Autodesk Inventor part; units mm, degrees
ref_plane "YZ Plane" through (0, 0, 0) normal (1, 0, 0) x (0, 1, 0)
ref_plane "XZ Plane" through (0, 0, 0) normal (0, 1, 0) x (-1, 0, 0)
ref_plane "XY Plane" through (0, 0, 0) normal (0, 0, 1) x (1, 0, 0)
sketch "Sketch1" plane through (0, 0, 0) normal (0, 1, 0) x (-1, 0, 0)
  line L0 (0, 0) -> (-70, 0)
  line L1 (-70, 0) -> (-70, -50)
  line L2 (-70, -50) -> (0, -50)
  line L3 (0, -50) -> (0, 0)
  line L4 (0, -50) -> (0, -67.7966)
  line L5 (0, -67.7966) -> (-70, -50)
  dimension "d0" = 70
  dimension "d1" = 50
  dimension "d45" = 14.264
extrude "Extrusion1" add sketch "Sketch1" along normal blind 6
sketch "Sketch2" plane through (0, 6, 0) normal (0, 1, 0) x (1, 0, 0)
  line L0 (70, 50) -> (58.37, 52.9568) construction
  line L1 (70, 50) -> (0, 67.7966) construction
  line L2 (58.37, 52.9568) -> (52.555, 54.4352)
  line L3 (52.555, 54.4352) -> (53.2942, 57.3427)
  line L4 (53.2942, 57.3427) -> (59.1092, 55.8643)
  line L5 (59.1092, 55.8643) -> (58.37, 52.9568)
  line L6 (23.4799, 61.8271) -> (17.6649, 63.3055)
  line L7 (17.6649, 63.3055) -> (18.4041, 66.213)
  line L8 (18.4041, 66.213) -> (24.2191, 64.7346)
  line L9 (24.2191, 64.7346) -> (23.4799, 61.8271)
  point P0 (0, 0)
  dimension "d9" = 12
  dimension "d10" = 6
  dimension "d11" = 3
  dimension "d15" = 6
  dimension "d16" = 3
  dimension "d17" = 30
extrude "Extrusion2" add sketch "Sketch2" against normal blind 6
sketch "Sketch3" plane through (0, 6, 0) normal (0, 1, 0) x (1, 0, 0)
  line L0 (70, 0) -> (70, 50)
  line L1 (70, 54) -> (64, 54)
  line L2 (64, 54) -> (64, 41)
  line L3 (64, 41) -> (70, 41)
  line L4 (70, 41) -> (70, 54)
  line L5 (70, 0) -> (64, 0)
  line L6 (64, 0) -> (64, 9)
  line L7 (64, 9) -> (70, 9)
  line L8 (70, 9) -> (70, 0)
  line L9 (70, 35) -> (64, 35)
  line L10 (64, 35) -> (64, 15)
  line L11 (64, 15) -> (70, 15)
  line L12 (70, 15) -> (70, 35)
  point P0 (0, 0)
  dimension "d18" = 6
  dimension "d20" = 6
  dimension "d21" = 9
  dimension "d22" = 6
  dimension "d23" = 6
  dimension "d27" = 20
  dimension "d36" = 13
extrude "Extrusion3" cut sketch "Sketch3" along normal through all both and the other way through all
sketch "Sketch4" plane through (0, 6, 0) normal (0, 1, 0) x (1, 0, 0)
  line L0 (64, 0) -> (64, 9)
  line L1 (64, 6.25) -> (56, 6.25)
  line L2 (49, 6.25) -> (49, 3.75)
  line L3 (49, 3.75) -> (53.7, 3.75)
  line L4 (64, 3.75) -> (64, 6.25)
  line L5 (64, 9) -> (70, 9)
  line L6 (64, 43.75) -> (56, 43.75)
  line L7 (49, 43.75) -> (49, 46.25)
  line L8 (49, 46.25) -> (53.7, 46.25)
  line L9 (64, 46.25) -> (64, 43.75)
  line L10 (70, 41) -> (64, 41)
  line L11 (64, 41) -> (64, 51.5254)
  line L12 (56, 47.7) -> (53.7, 47.7)
  line L13 (53.7, 47.7) -> (53.7, 46.25)
  line L14 (53.7, 42.3) -> (56, 42.3)
  line L15 (56, 42.3) -> (56, 43.75)
  line L16 (53.7, 7.7) -> (56, 7.7)
  line L17 (56, 7.7) -> (56, 6.25)
  line L18 (56, 2.3) -> (53.7, 2.3)
  line L19 (53.7, 2.3) -> (53.7, 3.75)
  line L20 (53.7, 6.25) -> (53.7, 7.7)
  line L21 (53.7, 3.75) -> (53.7, 6.25) construction
  line L22 (56, 6.25) -> (56, 3.75) construction
  line L23 (56, 3.75) -> (56, 2.3)
  line L24 (56, 3.75) -> (64, 3.75)
  line L25 (53.7, 3.75) -> (56, 3.75) construction
  line L26 (56, 6.25) -> (53.7, 6.25) construction
  line L27 (53.7, 6.25) -> (49, 6.25)
  line L28 (53.7, 43.75) -> (53.7, 42.3)
  line L29 (53.7, 46.25) -> (53.7, 43.75) construction
  line L30 (53.7, 43.75) -> (49, 43.75)
  line L31 (56, 43.75) -> (53.7, 43.75) construction
  line L32 (56, 46.25) -> (56, 47.7)
  line L33 (56, 43.75) -> (56, 46.25) construction
  line L34 (53.7, 46.25) -> (56, 46.25) construction
  line L35 (56, 46.25) -> (64, 46.25)
  line L36 (6, 10) -> (12, 10)
  line L37 (12, 10) -> (12, 16)
  line L38 (12, 16) -> (6, 16)
  line L39 (6, 16) -> (6, 10)
  line L40 (6, 31) -> (12, 31)
  line L41 (12, 31) -> (12, 37)
  line L42 (12, 37) -> (6, 37)
  line L43 (6, 37) -> (6, 31)
  line L44 (0, 0) -> (64, 0)
  line L45 (0, 67.7966) -> (0, 0)
  point P0 (64, 45)
  dimension "d37" = 15
  dimension "d38" = 2.5
  dimension "d42" = 15
  dimension "d43" = 2.5
  dimension "d44" = 2.75
  dimension "d46" = 2.75
  dimension "d47" = 5.4
  dimension "d48" = 2.3
  dimension "d49" = 5.4
  dimension "d50" = 8
  dimension "d51" = 8
  dimension "d52" = 6
  dimension "d53" = 6
  dimension "d54" = 6
  dimension "d55" = 6
  dimension "d56" = 10
  dimension "d57" = 6
  dimension "d58" = 15
extrude "Extrusion4" cut sketch "Sketch4" along normal through all both and the other way through all
equation "\"d15\" = d10"
equation "\"d16\" = d11"
equation "\"d18\" = d20"
equation "\"d42\" = d37"
equation "\"d43\" = d38"
equation "\"d44\" = d46"
equation "\"d50\" = d51"
equation "\"d54\" = d52"
properties part number "pinball-case-left-wal-scaledl"
Geometry: final body of the model. Coordinates: model frame, mm. A direction names the side the tool comes from. Give positions to 0.01 mm unless a question says otherwise; leave off trailing zeros. Loops run counter-clockwise (first coordinate to the right, second up) from the corner with the lowest first, then second, coordinate; pieces in that order, holes last. Notation, with made-up numbers: (-12, -20.75) - (12, -20.75) arc R23 ccw to (12, 0.25) - close; hole circle Ø5 at (55, 28.25). An arc over 180 degrees is marked (long way). One line per question, with ' | ' between items. Start each with the question number.
(1) Reachability of faces 1 (the flat face through (6, 3, -34)), 2 (the flat face through (64, 3, -8)), 3 (the flat face through (64, 3, -25)), 4 (the flat face through (64, 3, -49)), 5 (the flat face through (8.709, 2.958, -65.582)) from +Z, -Z, +X, -X, +Y, -Y: full face, straight path, thin tool, end or side. Return the list, or none.
(2) Section query B-B on x = 7.5. Return loops of the section in (y, z), then the cut area to 3 significant figures.
(3) Section query C-C on z = -23.5. Return loops of the section in (x, y), then the cut area to 3 significant figures.
(4) Section query D-D on y = 2.65. Count the separate pieces of the cut face and the enclosed holes in it, then the cut area to 3 significant figures.
(5) Contact query for flat-ended pins moving along their axis: pin 1 (2 mm diameter, centred on y = 3.5, z = -45.5, fed in from +X); pin 2 (3 mm diameter, centred on x = 66, y = 3.5, fed in from -Z); pin 3 (1 mm diameter, centred on y = 4, z = -30, fed in from -X); pin 4 (1.8 mm diameter, centred on x = 8.5, y = 4.5, fed in from -Z). Output: stop coordinate, or through.
(6) Ray query, line 1 (Z direction, x = 61.5, y = 1.6); line 2 (Z direction, x = 50.5, y = 4.4); line 3 (X direction, y = 1.35, z = -36.5). Return the intervals inside material, ascending. Write a range as from..to.
(7) Section query A-A on x = 65. Return loops of the section in (y, z).
The answers:
1) face 1: +Y, -Y | face 2: +Z, +X, +Y, -Y | face 3: +X, +Y, -Y | face 4: -Z, +X, +Y, -Y | face 5: -Z, +Y, -Y
2) outline: (0, -65.89) - (6, -65.89) - (6, -37) - (0, -37) - close; (0, -31) - (6, -31) - (6, -16) - (0, -16) - close; (0, -10) - (6, -10) - (6, 0) - (0, 0) - close | area: 323 mm2
3) outline: (0, 0) - (64, 0) - (64, 6) - (0, 6) - close | area: 384 mm2
4) separate pieces: 1 | enclosed holes: 2 | area: 3,770 mm2
5) pin 1: x = 64 | pin 2: z = -41 | pin 3: x = 0 | pin 4: z = -65.86
6) line 1: -52.16..-46.25, -43.75..-6.25, -3.75..0 | line 2: -54.96..-46.25, -43.75..-6.25, -3.75..0 | line 3: 0..6, 12..70
7) outline: (0, -41) - (6, -41) - (6, -35) - (0, -35) - close; (0, -15) - (6, -15) - (6, -9) - (0, -9) - close
